```python
from build123d import *

# Parameters (mm, degrees)
BOSS_EXTRUDE1_DEPTH = 14.605
FILLET1_R           = 6.35
CUT_EXTRUDE1_DEPTH  = 12.7
SKETCH5_W           = 290.733643468
SKETCH5_H           = 157.6979616
BOSS_EXTRUDE2_DEPTH = 1.905
FILLET2_R           = 2.54


with BuildPart() as part:
    # Sketch1 → Boss-Extrude1 (new body)
    with BuildSketch(Plane(origin=(0, 0, 0), x_dir=(1, 0, 0), z_dir=(0, 1, 0))):
        with BuildLine():
            Line((-150.5839, -100.33), (150.5839, -100.33))
            ThreePointArc((150.5839, -100.33), (161.072839149, -95.985339149), (165.4175, -85.4964))
            Line((165.4175, -85.4964), (165.4175, 85.4964))
            ThreePointArc((165.4175, 85.4964), (161.072839149, 95.985339149), (150.5839, 100.33))
            Line((150.5839, 100.33), (-150.5839, 100.33))
            ThreePointArc((-150.5839, 100.33), (-161.072839149, 95.985339149), (-165.4175, 85.4964))
            Line((-165.4175, 85.4964), (-165.4175, -85.4964))
            ThreePointArc((-165.4175, -85.4964), (-161.072839149, -95.985339149), (-150.5839, -100.33))
        make_face()
    extrude(amount=BOSS_EXTRUDE1_DEPTH)

    # Fillet1
    fillet1_edges = [part.edges().sort_by_distance(p)[0] for p in [
        (161.072839149, 14.605, -95.985339149),
        (0, 14.605, -100.33),
        (-161.072839149, 14.605, -95.985339149),
        (-165.4175, 14.605, 0),
        (-161.072839149, 14.605, 95.985339149),
        (0, 14.605, 100.33),
        (161.072839149, 14.605, 95.985339149),
        (165.4175, 14.605, 0),
    ]]
    fillet(fillet1_edges, radius=FILLET1_R)

    # Sketch2 → Cut-Extrude1 (cut)
    with BuildSketch(Plane.XZ):
        with BuildLine():
            Line((-148.6789, -98.425), (148.6789, -98.425))
            ThreePointArc((148.6789, -98.425), (159.167839149, -94.080339149), (163.5125, -83.5914))
            Line((163.5125, -83.5914), (163.5125, 83.5914))
            ThreePointArc((163.5125, 83.5914), (159.167839149, 94.080339149), (148.6789, 98.425))
            Line((148.6789, 98.425), (-148.6789, 98.425))
            ThreePointArc((-148.6789, 98.425), (-159.167839149, 94.080339149), (-163.5125, 83.5914))
            Line((-163.5125, 83.5914), (-163.5125, -83.5914))
            ThreePointArc((-163.5125, -83.5914), (-159.167839149, -94.080339149), (-148.6789, -98.425))
        make_face()
    extrude(amount=-CUT_EXTRUDE1_DEPTH, mode=Mode.SUBTRACT)

    # Sketch3 → Cut-Loft1 section 0
    with BuildSketch(Plane(origin=(0, 14.605, 0), x_dir=(1, 0, 0), z_dir=(0, 1, 0))):
        with BuildLine():
            Line((-142.875, -76.2), (142.875, -76.2))
            Line((142.875, -76.2), (142.875, 76.2))
            Line((142.875, 76.2), (-142.875, 76.2))
            Line((-142.875, 76.2), (-142.875, -76.2))
        make_face()
    # Sketch4 → Cut-Loft1 section 1
    with BuildSketch(Plane(origin=(0, 10.16, 0), x_dir=(1, 0, 0), z_dir=(0, 1, 0))):
        with BuildLine():
            Line((-139.7, -73.025), (139.7, -73.025))
            Line((139.7, -73.025), (139.7, 73.025))
            Line((139.7, 73.025), (-139.7, 73.025))
            Line((-139.7, 73.025), (-139.7, -73.025))
        make_face()
    loft(mode=Mode.SUBTRACT)

    # Sketch5 → Boss-Extrude2 (add)
    with BuildSketch(Plane.XZ.offset(-12.7)):
        Rectangle(SKETCH5_W, SKETCH5_H)
    extrude(amount=BOSS_EXTRUDE2_DEPTH)

    # Fillet2
    # the kernel refuses this fillet: 2.54 mm, written as the material it takes off along each edge
    with BuildSketch(Plane(origin=(151.515182796, 10.795, -78.8489808), x_dir=(0, 1, 0), z_dir=(-1, 0, 0)), Plane(origin=(-151.515182796, 10.795, 78.8489808), x_dir=(0, 1, 0), z_dir=(1, 0, 0))) as fillet2_piece_1:
        with BuildLine():
            CenterArc((2.54, -2.459344425), FILLET2_R, 104.477512186, 75.522487814)
            Line((0, -2.459344425), (-0.0508, -2.459344425))
            Line((-0.0508, -2.459344425), (-0.0508, 0))
            Line((-0.0508, 0), (0, 0.0508))
            ThreePointArc((0, 0.0508), (0.9525, 0.0508), (1.8923, 0.049186888))
            Line((1.8923, 0.049186888), (1.905, 0))
        make_face()
    extrude(amount=303.030365593, mode=Mode.SUBTRACT)
    with BuildSketch(Plane(origin=(-145.366821734, 10.795, -84.997341863), x_dir=(0, 1, 0), z_dir=(0, 0, 1)), Plane(origin=(145.366821734, 10.795, 84.997341863), x_dir=(0, 1, 0), z_dir=(0, 0, -1))) as fillet2_piece_2:
        with BuildLine():
            CenterArc((2.54, -2.459344425), FILLET2_R, 104.477512186, 75.522487814)
            Line((0, -2.459344425), (-0.0508, -2.459344425))
            Line((-0.0508, -2.459344425), (-0.0508, 0))
            Line((-0.0508, 0), (0, 0.0508))
            ThreePointArc((0, 0.0508), (0.9525, 0.0508), (1.8923, 0.049186888))
            Line((1.8923, 0.049186888), (1.905, 0))
        make_face()
    extrude(amount=169.994683725, mode=Mode.SUBTRACT)


solid = part.part
```
Input: part model. Units: mm. Frame: model coordinates. A direction names the side the tool comes from. Coordinates: 2 decimals unless noted, no trailing zeros.
Q1. Contact query for flat-ended pins moving along their axis: pin 1 (2 mm diameter, centred on x = -19.5, y = 11.5, fed in from +Z); pin 2 (8 mm diameter, centred on x = 97, z = 17.5, fed in from -Y) (3 decimals); pin 3 (10 mm diameter, centred on x = 32, z = -56.5, fed in from +Y). Output: stop coordinate, or through.
Results are:
pin 1: stops at z = 99.92
pin 2: stops at y = 10.795
pin 3: stops at y = 12.7
Q2. Line query: line 1 along Z through (x, y) = (-34.5, 5.25) (3 decimals); line 2 along Z through (x, y) = (-110, 11) (3 decimals); line 3 along X through (y, z) = (8, 2). Output: solid intervals per line, ascending.
Results are:
line 1: z = -100.33 to -98.425, 98.425 to 100.33
line 2: z = -99.706 to -98.425, -77.389 to 77.389, 98.425 to 99.706
line 3: x = -165.42 to -163.51, 163.51 to 165.42
Q3. Set-up query: faces 4 (the cylindrical face through (159.052, 6.261, -94.195)), 5 (the cylindrical face through (-2.1, 13.4, -97.7)). Return all of +Z, -Z, +X, -X, +Y, -Y with unobstructed straight access to the full face (end or side cutting, diameter ignored); none if empty.
Results are:
face 4: -Y
face 5: -Z, +X, -X, +Y
Q4. Mould query, pull axis X, two halves, no side actions, for faces 1 (the flat face through (2, 4, -100.33)), 2 (the flat face through (-2, 12.7, 1)), 3 (the cylindrical face through (160.957, 4.07, 96.1)). Classes: +X half, -X half, draft (parallel to the pull), parting line (faces both ways), or undercut.
Results are:
face 1: draft
face 2: undercut
face 3: +X half
